Geometry: final body of the model. Coordinates: model frame, mm. A direction names the side the tool comes from. Coordinates: 2 decimals unless noted, no trailing zeros. Order: outer loops, then holes, each group sorted by start corner. A loop starts at its lowest first (then second) coordinate and runs counter-clockwise, first axis right, second up. Notation, with made-up numbers: (-4, -24.75) -> (45, -24.75) arc R16 ccw to (45, -4.75) -> close; hole circle Ø8 at (48, 50.5). An arc over 180 degrees is marked (long way). Use one line per item in the form item = value.
```python
from build123d import *

# Parameters (mm, degrees)
F0_R     = 1.5875
F0_W     = 15.748
F0_H     = 23.368
F0_W_2   = 6.858
F0_H_2   = 6.35
F1_DEPTH = 5.715
F2_W     = 25.4
F2_H     = 33.02
F2_R     = 1.5875
F2_W_2   = 15.748
F2_H_2   = 23.368
F3_DEPTH = 1.27


with BuildPart() as f1:
    # F0 (on Top) → F1 (new body)
    with BuildSketch(Plane.XY):
        Polygon((12.7, 16.51), (-12.7, 16.51), (-12.7, 11.811), (-12.7, 5.461), (-12.7, -5.588), (-12.7, -11.938), (-12.7, -16.51), (12.7, -16.51), (12.7, -11.938), (12.7, -5.588), (12.7, 5.461), (12.7, 11.811), align=None)
        with Locations((0, -14.351)):
            Circle(F0_R, mode=Mode.SUBTRACT)
        Rectangle(F0_W, F0_H, mode=Mode.SUBTRACT)
        with Locations((0, 14.224)):
            Circle(F0_R, mode=Mode.SUBTRACT)
        with Locations((-16.129, 8.636)):
            Rectangle(F0_W_2, F0_H_2)
        with Locations((16.129, 8.636)):
            Rectangle(F0_W_2, F0_H_2)
        with Locations((-16.129, -8.763)):
            Rectangle(F0_W_2, F0_H_2)
        with Locations((16.129, -8.763)):
            Rectangle(F0_W_2, F0_H_2)
    extrude(amount=-F1_DEPTH)

    # F2 (on face) → F3 (join)
    with BuildSketch(Plane.XY):
        Rectangle(F2_W, F2_H)
        with Locations((0, -14.351)):
            Circle(F2_R, mode=Mode.SUBTRACT)
        with Locations((0, 14.224)):
            Circle(F2_R, mode=Mode.SUBTRACT)
        Rectangle(F2_W_2, F2_H_2, mode=Mode.SUBTRACT)
    extrude(amount=F3_DEPTH)


solid = f1.part
```
1) Section D-D, the plane z = -3.5. Output: boundary loops of the cut face in (x, y) (1 decimal).
Results found:
outline = (-19.6, -11.9) -> (-12.7, -11.9) -> (-12.7, -16.5) -> (12.7, -16.5) -> (12.7, -11.9) -> (19.6, -11.9) -> (19.6, -5.6) -> (12.7, -5.6) -> (12.7, 5.5) -> (19.6, 5.5) -> (19.6, 11.8) -> (12.7, 11.8) -> (12.7, 16.5) -> (-12.7, 16.5) -> (-12.7, 11.8) -> (-19.6, 11.8) -> (-19.6, 5.5) -> (-12.7, 5.5) -> (-12.7, -5.6) -> (-19.6, -5.6) -> close; hole (-7.9, -11.7) -> (7.9, -11.7) -> (7.9, 11.7) -> (-7.9, 11.7) -> close; hole circle Ø3.2 at (0, -14.4); hole circle Ø3.2 at (0, 14.2)
2) Section C-C, the plane y = -2. Output: boundary loops of the cut face in (x, z) (3 decimals).
Results found:
outline = (-12.7, -5.715) -> (-7.874, -5.715) -> (-7.874, 1.27) -> (-12.7, 1.27) -> close; (7.874, -5.715) -> (12.7, -5.715) -> (12.7, 1.27) -> (7.874, 1.27) -> close
3) Access query for faces 1 (the flat face through (16, 11.811, -3)), 2 (the flat face through (16, 5.461, -3)), 3 (the flat face through (-16, -11.938, -3)), 4 (the flat face through (-7.874, 0, -2)). Directions: +Z, -Z, +X, -X, +Y, -Y. A direction counts if a zero-diameter tool reaches every point of the face in a straight line with its end or side. Return the directions, or none.
Results found:
face_1 = +Z, -Z, +X, +Y
face_2 = +Z, -Z, +X
face_3 = +Z, -Z, -X, -Y
face_4 = +Z, -Z
4) Material intervals for probe 1 along Y at (x, z) = (0, -0.5); probe 2 along X at (y, z) = (-1.5, -3.5); probe 3 along Y at (x, z) = (-2.5, -1), sorted ascending. Write a range as from..to.
Results found:
probe_1 = -16.51..-15.94, -12.76..-11.68, 11.68..12.64, 15.81..16.51
probe_2 = -12.7..-7.87, 7.87..12.7
probe_3 = -16.51..-11.68, 11.68..16.51
5) Section B-B, the plane x = 17. Output: boundary loops of the cut face in (y, z) (3 decimals).
Results found:
outline = (-11.938, -5.715) -> (-5.588, -5.715) -> (-5.588, 0) -> (-11.938, 0) -> close; (5.461, -5.715) -> (11.811, -5.715) -> (11.811, 0) -> (5.461, 0) -> close
6) Contact query for flat-ended pins moving along their axis: P1, Ø1.9, axis at x = -17, y = -10, coming from the +Z side; P2, Ø2, axis at y = -0.5, z = -2, coming from the +X side; P3, Ø6, axis at x = 0, y = 6.5, coming from the +Z side; P4, Ø3, axis at x = 14.5, z = -1.5, coming from the +Y side. Output: stop coordinate, or through.
Results found:
P1 = 0
P2 = 12.7
P3 = through
P4 = 11.81
7) Pull-direction query (X, two-part tool) for faces 5 (the flat face through (19.558, 9, -3)), 6 (the flat face through (8.3, 0.2, 1.27)), 7 (the flat face through (0, 11.684, -2)); classes: released by +X, released by -X, zero draft, split by the parting line, or undercut.
Results found:
face_5 = released by +X
face_6 = zero draft
face_7 = undercut
8) Section A-A, the plane x = 0. Output: boundary loops of the cut face in (y, z) (1 decimal), and give its area (3 significant figures).
Results found:
outline = (-16.5, -5.7) -> (-15.9, -5.7) -> (-15.9, 1.3) -> (-16.5, 1.3) -> close; (-12.8, -5.7) -> (-11.7, -5.7) -> (-11.7, 1.3) -> (-12.8, 1.3) -> close; (11.7, -5.7) -> (12.6, -5.7) -> (12.6, 1.3) -> (11.7, 1.3) -> close; (15.8, -5.7) -> (16.5, -5.7) -> (16.5, 1.3) -> (15.8, 1.3) -> close
area = 23.1 mm2
